Check sheet for the modelled part. Datum: model origin and axes. Units: mm. A direction names the side the tool comes from. Give positions to 0.01 mm unless a question says otherwise; leave off trailing zeros. Order: outer loops, then holes, each group sorted by start corner. A loop starts at its lowest first (then second) coordinate and runs counter-clockwise, first axis right, second up. Notation, with made-up numbers: M 88.5,79 L 118.5,79 A26 ccw 118.5,109 Z; hole C 33.25,76.25 d4. An arc over 180 degrees is marked long. One line per question, with ' | ' between items. Start each with the question number.
Autodesk Inventor part; units mm, degrees
ref_plane "YZ Plane" through (0, 0, 0) normal (1, 0, 0) x (0, 1, 0)
ref_plane "XZ Plane" through (0, 0, 0) normal (0, 1, 0) x (-1, 0, 0)
ref_plane "XY Plane" through (0, 0, 0) normal (0, 0, 1) x (1, 0, 0)
ref_plane "作業平面1" through (0, 2, 0) normal (0, 1, 0) x (1, 0, 0)
sketch "スケッチ4" plane through (0, 2, 0) normal (0, 1, 0) x (1, 0, 0)
  line L0 (3, 73) -> (33, 73)
  line L1 (3, 73) -> (3, 23)
  line L2 (3, 20) -> (3, 3)
  line L3 (81, 3) -> (81, 33)
  line L4 (81, 33) -> (84, 33)
  line L5 (84, 33) -> (84, 3)
  line L6 (117, 3) -> (117, 18)
  line L7 (117, 18) -> (120, 18)
  line L8 (117, 28) -> (117, 35)
  line L9 (120, 28) -> (117, 28)
  line L10 (120, 28) -> (120, 38)
  line L11 (117, 38) -> (97, 38)
  line L12 (97, 38) -> (97, 45)
  line L13 (97, 45) -> (94, 45)
  line L14 (94, 45) -> (94, 35)
  line L15 (94, 35) -> (117, 35)
  line L16 (97, 73) -> (97, 66)
  line L17 (97, 66) -> (94, 66)
  line L18 (94, 66) -> (94, 73)
  line L19 (33, 73) -> (33, 23)
  line L20 (33, 23) -> (13, 23)
  line L21 (13, 23) -> (13, 20)
  line L22 (13, 20) -> (36, 20)
  line L23 (36, 20) -> (36, 73)
  line L24 (36, 73) -> (46, 73)
  line L25 (46, 73) -> (46, 20)
  line L26 (46, 20) -> (49, 20)
  line L27 (49, 20) -> (49, 73)
  line L28 (117, 38) -> (117, 40.5)
  line L29 (117, 40.5) -> (120, 40.5)
  line L30 (120, 40.5) -> (120, 38)
  line L31 (117, 73) -> (117, 70.5)
  line L32 (117, 70.5) -> (120, 70.5)
  line L33 (0, 0) -> (0, 76)
  line L34 (0, 76) -> (120, 76)
  line L35 (120, 76) -> (120, 70.5)
  line L36 (0, 0) -> (120, 0)
  line L37 (120, 0) -> (120, 18)
  line L38 (3, 23) -> (3, 20)
  line L39 (33, 3) -> (33, 11)
  line L40 (33, 11) -> (36, 11)
  line L41 (36, 11) -> (36, 3)
  line L42 (3, 3) -> (33, 3)
  line L43 (36, 3) -> (81, 3)
  line L44 (94, 3) -> (94, 13)
  line L45 (94, 13) -> (97, 13)
  line L46 (97, 13) -> (97, 3)
  line L47 (84, 3) -> (94, 3)
  line L48 (97, 3) -> (117, 3)
  line L49 (117, 73) -> (97, 73)
  line L50 (94, 73) -> (49, 73)
  dimension "d29" = 3
  dimension "d30" = 30
  dimension "d34" = 3
  dimension "d35" = 20
  dimension "d36" = 3
  dimension "d37" = 10
  dimension "d39" = 3
  dimension "d41" = 32
  dimension "d42" = 3
  dimension "d60" = 3
  dimension "d61" = 3
  dimension "d63" = 7
  dimension "d64" = 7
  dimension "d65" = 15
  dimension "d66" = 10
  dimension "d67" = 2.5
  dimension "d68" = 3
  dimension "d69" = 3
  dimension "d70" = 2.5
  dimension "d75" = 76
  dimension "d78" = 3
  dimension "d79" = 3
  dimension "d80" = 3
  dimension "d81" = 20
  dimension "d82" = 50
  dimension "d84" = 120
  dimension "d85" = 3
  dimension "d86" = 8
  dimension "d87" = 3
  dimension "d88" = 30
  dimension "d89" = 3
  dimension "d90" = 10
  dimension "d91" = 10
  dimension "d92" = 35
extrude "押し出し5" add sketch "スケッチ4" along normal blind 5
sketch "スケッチ6" plane through (0, 2, 0) normal (0, 1, 0) x (1, 0, 0)
  line L0 (0, 0) -> (120, 0)
  line L1 (0, 0) -> (120, 0)
  line L2 (120, 18) -> (117, 18)
  line L3 (120, 0) -> (120, 18)
  line L4 (120, 18) -> (117, 18)
  line L5 (117, 18) -> (117, 3)
  line L6 (117, 18) -> (117, 3)
  line L7 (3, 3) -> (3, 73)
  line L8 (117, 3) -> (3, 3)
  line L9 (3, 3) -> (3, 73)
  line L10 (97, 73) -> (117, 73)
  line L11 (3, 73) -> (117, 73)
  line L12 (117, 73) -> (117, 70.5)
  line L13 (117, 73) -> (117, 70.5)
  line L14 (117, 70.5) -> (120, 70.5)
  line L15 (117, 70.5) -> (120, 70.5)
  line L16 (120, 70.5) -> (120, 76)
  line L17 (120, 70.5) -> (120, 76)
  line L18 (120, 76) -> (0, 76)
  line L19 (120, 76) -> (0, 76)
  line L20 (0, 76) -> (0, 0)
  line L21 (0, 76) -> (0, 0)
  line L22 (120, 28) -> (117, 28)
  line L23 (117, 28) -> (120, 28)
  line L24 (120, 40.5) -> (120, 28)
  line L25 (120, 28) -> (120, 40.5)
  line L26 (117, 40.5) -> (120, 40.5)
  line L27 (120, 40.5) -> (117, 40.5)
  line L28 (117, 40.5) -> (117, 28)
extrude "押し出し6" add sketch "スケッチ6" along normal blind 6.5
sketch "スケッチ7" plane through (0, 2, 0) normal (0, 1, 0) x (1, 0, 0)
  line L0 (0, 0) -> (120, 0)
  line L1 (120, 70.5) -> (120, 76)
  line L2 (0, 0) -> (120, 0)
  line L3 (120, 0) -> (120, 76)
  line L4 (120, 76) -> (0, 76)
  line L5 (0, 76) -> (0, 0)
extrude "押し出し7" add sketch "スケッチ7" against normal blind 1.5
properties part number "BASE_revised"
Item 1: Section check D-D, the plane x = 26. Record the cut outline in (y, z), then the cut area to 3 significant figures.
Item 2: Set-up check for faces 1 (the face through (118, 5, -70.5)), 2 (the face through (34, 7, -7)): record each of +Z, -Z, +X, -X, +Y, -Y from which the full face is reachable in a straight line by a thin tool's end or side.
Item 3: Section check A-A, the plane z = -50. Record the cut outline in (x, y).
Item 4: Draft check along Z on faces 3 (the face through (95, 4, -13)), 4 (the face through (59, 5, 0)). Enter one of: released by +Z, released by -Z, zero draft, split by the parting line, or undercut.
Item 5: Scan lines: probe 1 along Z at (x, y) = (28, 3.75); probe 2 along X at (y, z) = (6.25, -46); probe 3 along X at (y, z) = (6.25, -69). Record each from-to range of solid material in increasing order. Write a range as [from, to].
Item 6: Section check C-C, the plane z = -6.5. Record the cut outline in (x, y).
Item 7: Go/stop test with flat-tipped pins: P1, Ø3, axis at x = 56.5, z = -55.5, coming from the +Y side; P2, Ø2.5, axis at y = 4.5, z = -43.5, coming from the +X side; P3, Ø1.5, axis at x = 36.5, z = -26, coming from the +Y side. Record where each tip stops, or that it passes through.
Item 8: Section check B-B, the plane x = 79. Record the cut outline in (y, z), then the cut area to 3 significant figures.
Reported:
1) outline: M 0.5,-76 L 8.5,-76 L 8.5,-73 L 2,-73 L 2,-23 L 7,-23 L 7,-20 L 2,-20 L 2,-3 L 8.5,-3 L 8.5,0 L 0.5,0 Z | area: 168 mm^2
2) face 1: +X, +Y | face 2: +Y
3) outline: M 0,0.5 L 120,0.5 L 120,2 L 49,2 L 49,7 L 46,7 L 46,2 L 36,2 L 36,7 L 33,7 L 33,2 L 3,2 L 3,8.5 L 0,8.5 Z
4) face 3: undercut | face 4: released by +Z
5) probe 1: z = [-76, -73], [-23, -20], [-3, 0] | probe 2: x = [0, 3], [33, 36], [46, 49] | probe 3: x = [0, 3], [33, 36], [46, 49], [94, 97]
6) outline: M 0,0.5 L 120,0.5 L 120,8.5 L 117,8.5 L 117,2 L 97,2 L 97,7 L 94,7 L 94,2 L 84,2 L 84,7 L 81,7 L 81,2 L 36,2 L 36,7 L 33,7 L 33,2 L 3,2 L 3,8.5 L 0,8.5 Z
7) P1: stops at y = 2 | P2: stops at x = 97 | P3: stops at y = 7
8) outline: M 0.5,-76 L 8.5,-76 L 8.5,-73 L 2,-73 L 2,-3 L 8.5,-3 L 8.5,0 L 0.5,0 Z | area: 153 mm^2
